Can you work these out from the model? Positions are in its coordinate system, mm. Give positions to 0.01 mm unless a question says otherwise; leave off trailing zeros. Loops run counter-clockwise (first coordinate to the right, second up) from the corner with the lowest first, then second, coordinate; pieces in that order, holes last. Notation, with made-up numbers: M -9.75,53.25 L 11.25,53.25 A19 ccw 11.25,85.25 Z; hole C 44.25,37 d6. An arc over 180 degrees is marked long. One line per item, written item: value. Start each with the question number.
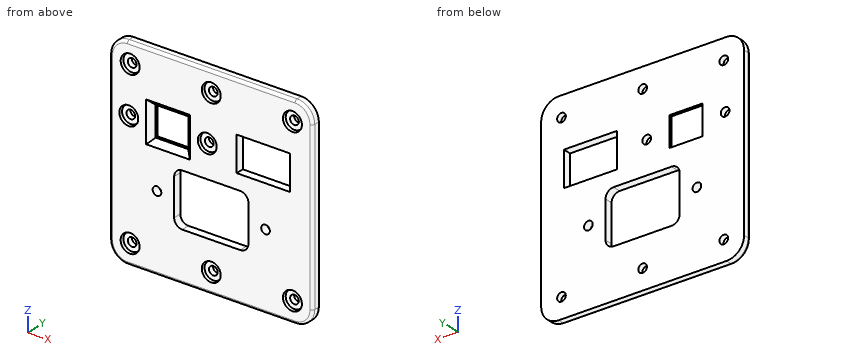
from build123d import *

# Parameters (mm, degrees)
F0_R     = 1.6
F0_W     = 12.1
F0_H     = 11
F0_W_2   = 19.7
F0_H_2   = 12.9
F1_DEPTH = 3
F2_R     = 3.5
F3_DEPTH = 1
F3_TAPER = 15
F4_R     = 1
F5_SIZE  = 2


with BuildPart() as f1:
    # F0 (on Front) → F1 (new body)
    with BuildSketch(Plane.XZ):
        with BuildLine():
            Line((68.5, 75), (6.5, 75))
            ThreePointArc((6.5, 75), (1.9038059223, 73.0961940777), (0, 68.5))
            Line((0, 68.5), (0, 6.5))
            ThreePointArc((0, 6.5), (1.9038059223, 1.9038059223), (6.5, 0))
            Line((6.5, 0), (68.5, 0))
            ThreePointArc((68.5, 0), (73.0961940777, 1.9038059223), (75, 6.5))
            Line((75, 6.5), (75, 68.5))
            ThreePointArc((75, 68.5), (73.0961940777, 73.0961940777), (68.5, 75))
        make_face()
        with Locations((7.5, 7.5)):
            Circle(F0_R, mode=Mode.SUBTRACT)
        with Locations((17.435, 28.1759891631)):
            Circle(F0_R, mode=Mode.SUBTRACT)
        with Locations((37.5, 7.5)):
            Circle(F0_R, mode=Mode.SUBTRACT)
        with Locations((67.5, 7.5)):
            Circle(F0_R, mode=Mode.SUBTRACT)
        with BuildLine():
            Line((26.785, 38.0809891631), (48.215, 38.0809891631))
            ThreePointArc((48.215, 38.0809891631), (50.3363203436, 37.2023095066), (51.215, 35.0809891631))
            Line((51.215, 35.0809891631), (51.215, 21.2709891631))
            ThreePointArc((51.215, 21.2709891631), (50.3363203436, 19.1496688195), (48.215, 18.2709891631))
            Line((48.215, 18.2709891631), (26.785, 18.2709891631))
            ThreePointArc((26.785, 18.2709891631), (24.6636796564, 19.1496688195), (23.785, 21.2709891631))
            Line((23.785, 21.2709891631), (23.785, 35.0809891631))
            ThreePointArc((23.785, 35.0809891631), (24.6636796564, 37.2023095066), (26.785, 38.0809891631))
        make_face(mode=Mode.SUBTRACT)
        with Locations((57.565, 28.1759891631)):
            Circle(F0_R, mode=Mode.SUBTRACT)
        with Locations((7, 50.0734709203)):
            Circle(F0_R, mode=Mode.SUBTRACT)
        with Locations((21.5, 50.0734709203)):
            Rectangle(F0_W, F0_H, mode=Mode.SUBTRACT)
        with Locations((36, 50.0734709203)):
            Circle(F0_R, mode=Mode.SUBTRACT)
        with Locations((7.5, 67.5)):
            Circle(F0_R, mode=Mode.SUBTRACT)
        with Locations((56.75, 50.0734709203)):
            Rectangle(F0_W_2, F0_H_2, mode=Mode.SUBTRACT)
        with Locations((37.5, 67.5)):
            Circle(F0_R, mode=Mode.SUBTRACT)
        with Locations((67.5, 67.5)):
            Circle(F0_R, mode=Mode.SUBTRACT)
    extrude(amount=F1_DEPTH)

    # F2 (on face) → F3 (cut)
    with BuildSketch(Plane.XZ.offset(3)):
        with Locations((7.5, 67.5)):
            Circle(F2_R)
        with Locations((37.5, 67.5)):
            Circle(F2_R)
        with Locations((67.5, 67.5)):
            Circle(F2_R)
        with Locations((36, 50.0734709203)):
            Circle(F2_R)
        with Locations((7, 50.0734709203)):
            Circle(F2_R)
        with Locations((67.5, 7.5)):
            Circle(F2_R)
        with Locations((37.5, 7.5)):
            Circle(F2_R)
        with Locations((7.5, 7.5)):
            Circle(F2_R)
    extrude(amount=-F3_DEPTH, taper=F3_TAPER, mode=Mode.SUBTRACT)

    # F4
    f4_edges = [f1.edges().sort_by_distance(p)[0] for p in [
        (37.5, -3, 0),
    ]]
    fillet(f4_edges, radius=F4_R)

    # F5
    f5_edges = [f1.edges().sort_by_distance(p)[0] for p in [
        (21.5, -3, 55.573471),
        (27.55, -3, 50.073471),
        (21.5, -3, 44.573471),
        (15.45, -3, 50.073471),
    ]]
    chamfer(f5_edges, length=F5_SIZE)


solid = f1.part
Q1. If we section it at C-C, the plane z = 32: Write out the boundary of the cut face in (x, y) (3 decimals).
Q2. If we section it at B-B, the plane x = 67.5: Write out the boundary of the cut face in (y, z), plus the area to 3 significant figures.
Q3. If we section it at D-D, the plane z = 67.5: Give the number of separate pieces and of enclosed holes in the cut face, plus the area to 3 significant figures.
Q4. I need wall thicknesses on line 1 along X through (y, z) = (-0.7, 7.5); line 2 along Z through (x, y) = (47, -0.75); line 3 along Z through (x, y) = (41, -1.35). Which ranges of each line are inside material? Lowest first, please.
Q5. If we section it at A-A, the plane x = 22: Write out the boundary of the cut face in (y, z), plus the area to 3 significant figures.
Q6. For P1, Ø4, axis at x = 57.56, z = 28.18, coming from the +Y side; P2, Ø4, axis at x = 7.5, z = 7.5, coming from the -Y side, each with a flat end and sliding along its axis, tell me the tip position at first contact or that it passes through.
Response:
1. outline: M 0,-2 A1 ccw 1,-3 L 23.785,-3 L 23.785,0 L 0,0 Z; M 51.215,-3 L 74,-3 A1 ccw 75,-2 L 75,0 L 51.215,0 Z
2. outline: M -3,1 A1 ccw -2,0 L 0,0 L 0,5.9 L -2,5.9 L -2,4.27 L -3,4 Z; M -3,11 L -2,10.73 L -2,9.1 L 0,9.1 L 0,65.9 L -2,65.9 L -2,64.27 L -3,64 Z; M -3,71 L -2,70.73 L -2,69.1 L 0,69.1 L 0,75 L -2,75 A1 ccw -3,74 Z
2. area: 198 mm^2
3. separate pieces: 4
3. enclosed holes: 0
3. area: 185 mm^2
4. line 1: 0 to 5.9, 9.1 to 35.9, 39.1 to 65.9, 69.1 to 75
4. line 2: 0 to 18.27, 38.08 to 43.62, 56.52 to 75
4. line 3: 0 to 18.27, 38.08 to 75
5. outline: M -3,1 A1 ccw -2,0 L 0,0 L 0,44.57 L -1,44.57 L -3,42.57 Z; M -3,57.57 L -1,55.57 L 0,55.57 L 0,75 L -2,75 A1 ccw -3,74 Z
5. area: 188 mm^2
6. P1: y = 0
6. P2: y = -2
